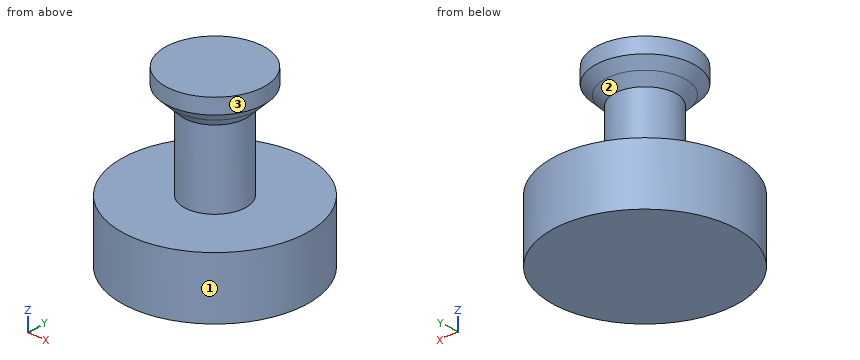
from build123d import *

# Parameters (mm, degrees)
F6_R      = 2.5
F7_DEPTH  = 12
F6_R_2    = 7.5
F8_DEPTH  = 5
F9_R      = 4
F9_R_2    = 2.5
F10_DEPTH = 2
F11_SIZE  = 0.74999


# Not quite as in the source:
# - a fillet or chamfer is up to 0.001 mm smaller than in the source, because OpenCascade refuses the exact size


with BuildPart() as f7:
    # F6 (on Top) → F7 (new body)
    with BuildSketch(Plane.XY):
        Circle(F6_R)
    extrude(amount=F7_DEPTH)

    # F6 (on Top) → F8 (join)
    with BuildSketch(Plane.XY):
        Circle(F6_R_2)
        Circle(F6_R, mode=Mode.SUBTRACT)
    extrude(amount=F8_DEPTH)

    # F9 (on face) → F10 (join)
    with BuildSketch(Plane.XY.offset(12)):
        Circle(F9_R)
        Circle(F9_R_2, mode=Mode.SUBTRACT)
        Circle(F9_R_2)
    extrude(amount=F10_DEPTH)

    # F11 (size 0.75 in the source; OpenCascade refuses exactly that, so slightly less here)
    f11_edges = [f7.edges().sort_by_distance(p)[0] for p in [
        (-4, 0, 12),
        (-2.5, 0, 12),
    ]]
    chamfer(f11_edges, length=F11_SIZE)


solid = f7.part
Verification items for the finished model (mm, model axes). Face numbers are marked on the shaded views. A direction names the side the tool comes from. Give positions to 0.01 mm unless a question says otherwise; leave off trailing zeros. Order: outer loops, then holes, each group sorted by start corner. A loop starts at its lowest first (then second) coordinate and runs counter-clockwise, first axis right, second up. Notation, with made-up numbers: M 86.25,-15.5 L 113.25,-15.5 A19 cw 113.25,5.5 Z; hole C -6,77 d3. An arc over 180 degrees is marked long. Use one line per item in the form item = value. Start each with the question number.
Q1. Go/stop test with flat-tipped pins: pin 1 Ø8 at (y, z) = (5.5, 12.5) entering from -X; pin 2 Ø6 at (x, z) = (-4.5, 8.5) entering from -Y; pin 3 Ø1 at (x, z) = (0.5, 7.5) entering from +Y. Record where each tip stops, or that it passes through.
Q2. Scan lines: line 1 along Z through (x, y) = (3.5, 4.25); line 2 along X through (y, z) = (0.5, 6.75); line 3 along Y through (x, z) = (1.5, 2.25). Record each from-to range of solid material in increasing order. Write a range as [from, to].
Q3. Access from +Z, -Z, +X, -X, +Y, -Y to the whole of each face (thin tool, end or side, straight path). Record for the marked faces 1, 2 and 3.
Q4. Section check C-C (z = 13.25). Enter the section's corners in (x, y), then the cut area to 3 significant figures.
Q5. Section check D-D (z = 8). Enter the section's corners in (x, y), then the cut area to 3 significant figures.
Evaluation:
q1.pin_1 = -3.7
q1.pin_2 = -2
q1.pin_3 = 2.5
q2.line_1 = [0, 5]
q2.line_2 = [-2.45, 2.45]
q2.line_3 = [-7.35, 7.35]
q3.face_1 = +Z, -Z
q3.face_2 = none
q3.face_3 = +Z
q4.outline = C 0,0 d8
q4.area = 50.3 mm2
q5.outline = C 0,0 d5
q5.area = 19.6 mm2
